Geometry check sheet. Reference: drawing and pictorial views, mm from the part's lowest x, y, z. Coordinates: 2 decimals unless noted, no trailing zeros. Loops run counter-clockwise (first coordinate to the right, second up) from the corner with the lowest first, then second, coordinate; pieces in that order, holes last. Notation, with made-up numbers: M -20.75,16.5 L -7.75,16.5 A21 cw -7.75,35.5 Z; hole C 19.5,39.5 d2. An arc over 180 degrees is marked long. Write each question's results on one line, items separated by ' | '. Start each with the question number.
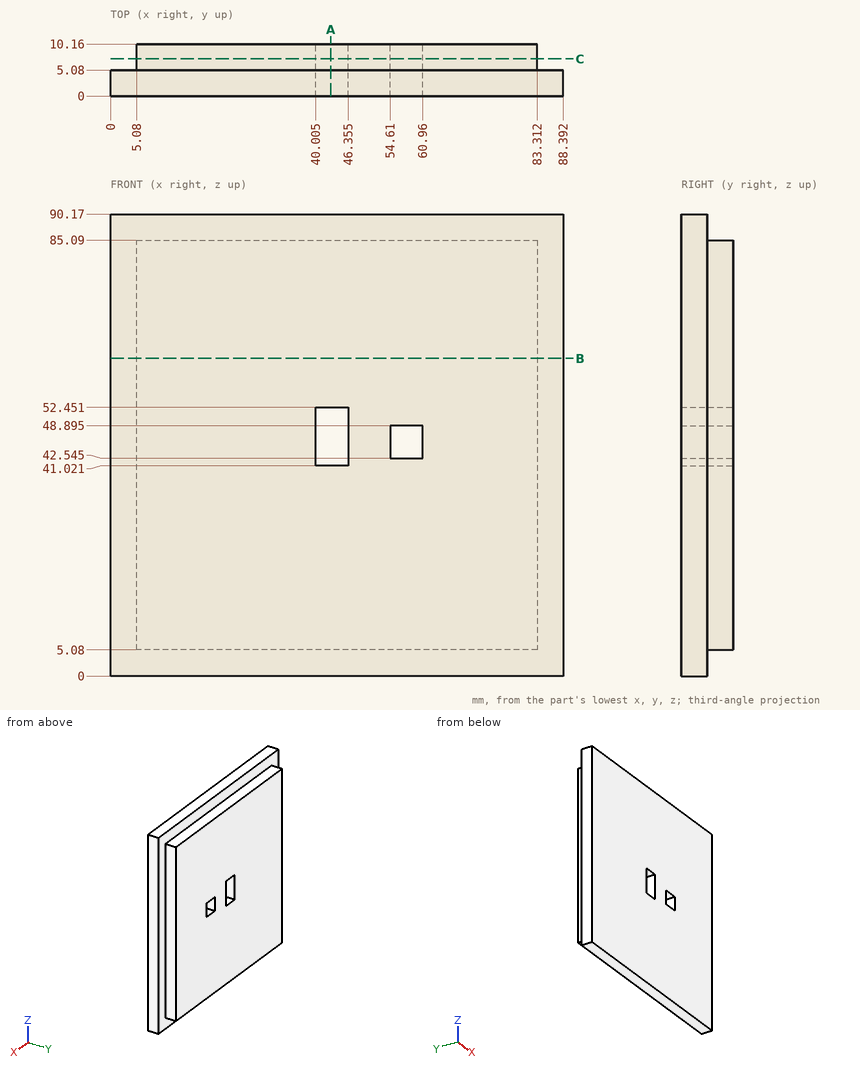
1) Gauge pin test, flat ends, axial feed: P1, Ø5, axis at y = 3, z = 45.5, coming from the -X side; P2, Ø5.5, axis at y = 9, z = 38, coming from the -X side; P3, Ø5, axis at y = 8, z = 11.5, coming from the +X side. Record the tip position at first contact, or that the pin passes through.
2) Section check B-B (z = 62). Enter the section's corners in (x, y).
3) Section check A-A (x = 43). Enter the section's corners in (y, z), then the cut area to 3 significant figures.
4) Thickness scan on probe 1 along X at (y, z) = (6.75, 43) (3 decimals); probe 2 along X at (y, z) = (8, 83); probe 3 along Z at (x, y) = (14.5, 8.25). Record the ranges inside material, lowest first.
5) Section check C-C (y = 7.25). Enter the section's corners in (x, z) (3 decimals), then the cut area to 3 significant figures.
Return value:
1) P1: stops at x = 0 | P2: stops at x = 5.08 | P3: stops at x = 83.31
2) outline: M 0,0 L 88.39,0 L 88.39,5.08 L 83.31,5.08 L 83.31,10.16 L 5.08,10.16 L 5.08,5.08 L 0,5.08 Z
3) outline: M 0,0 L 5.08,0 L 5.08,5.08 L 10.16,5.08 L 10.16,41.02 L 0,41.02 Z; M 0,52.45 L 10.16,52.45 L 10.16,85.09 L 5.08,85.09 L 5.08,90.17 L 0,90.17 Z | area: 748 mm2
4) probe 1: x = 5.08 to 40.005, 46.355 to 54.61, 60.96 to 83.312 | probe 2: x = 5.08 to 83.31 | probe 3: z = 5.08 to 85.09
5) outline: M 5.08,5.08 L 83.312,5.08 L 83.312,85.09 L 5.08,85.09 Z; hole M 40.005,41.021 L 46.355,41.021 L 46.355,52.451 L 40.005,52.451 Z; hole M 54.61,42.545 L 60.96,42.545 L 60.96,48.895 L 54.61,48.895 Z | area: 6,150 mm2
